Autodesk Inventor part; units mm, degrees
ref_plane "YZ Plane" through (0, 0, 0) normal (1, 0, 0) x (0, 1, 0)
ref_plane "XZ Plane" through (0, 0, 0) normal (0, 1, 0) x (-1, 0, 0)
ref_plane "XY Plane" through (0, 0, 0) normal (0, 0, 1) x (1, 0, 0)
sketch "Эскиз1" plane through (0, 0, 0) normal (0, 0, 1) x (1, 0, 0)
  line L0 (-17.6, 17.6) -> (17.6, 17.6)
  line L1 (17.6, 17.6) -> (17.6, -17.6)
  line L2 (17.6, -17.6) -> (-17.6, -17.6)
  line L3 (-17.6, -17.6) -> (-17.6, 17.6)
  point P0 (13, -13)
  point P1 (-13, -13)
  point P2 (13, 13)
  point P3 (-13, 13)
  dimension "d0" = 35.2
  dimension "d1" = 35.2
extrude "Выдавливание1" add sketch "Эскиз1" along normal blind 26
sketch "Эскиз2" plane through (0, 0, 26) normal (0, 0, 1) x (1, 0, 0)
  circle A0 centre (0, 0) radius 11
  dimension "d6" = 22
extrude "Выдавливание2" add sketch "Эскиз2" along normal blind 2
sketch "Эскиз3" plane through (0, 0, 28) normal (0, 0, 1) x (1, 0, 0)
  circle A0 centre (0, 0) radius 11
  circle A1 centre (0, 0) radius 2.5
  dimension "d9" = 5
extrude "Выдавливание3" add sketch "Эскиз3" along normal blind 22 contours A1
sketch "Эскиз4" plane through (0, 0, 50) normal (0, 0, 1) x (1, 0, 0)
  line L0 (0, 2) -> (3.1194, 2)
  line L1 (3.1194, 2) -> (3.1194, 3.4913)
  line L2 (3.1194, 3.4913) -> (-4.7004, 3.4913)
  line L3 (-4.7004, 3.4913) -> (-4.7004, 2)
  line L4 (-4.7004, 2) -> (0, 2)
extrude "Выдавливание4" cut sketch "Эскиз4" against normal blind 15
hole "Отверстие1" at (13, -13, 0) at (13, 13, 0) at (-13, 13, 0) at (-13, -13, 0) direction (0, 0, 1) diameter 3 end through all
fillet "Сопряжение1" radius 1 4 edges at (-17.6, -17.6, 13) (17.6, -17.6, 13) (17.6, 17.6, 13) (-17.6, 17.6, 13)
properties part number "MotorNema14"
The model under review builds one solid part; all positions refer to its coordinate system, in mm. A direction names the side the tool comes from. Give positions to 0.01 mm unless a question says otherwise; leave off trailing zeros. Write each loop counter-clockwise with the first axis right and the second up, starting at its lowest first coordinate (ties: lowest second). Pieces come first, ordered by that corner, then holes. Notation, with made-up numbers: M -20,59.5 L -6,59.5 A20 ccw -6,91.5 Z; hole C -23.5,17 d8. An arc over 180 degrees is marked long. Write each question's results on one line, items separated by ' | '. Start each with the question number.
1. We need section D-D (y = 0). Write out the cut boundary in (x, z), and give its area (3 significant figures).
2. We need section A-A (x = 13). Write out the cut boundary in (y, z).
3. For probe 1 along Y at (x, z) = (13, 17); probe 2 along Z at (x, y) = (-15, 13.5), list the stretches that pass through material, from the lowest coordinate up. Write a range as [from, to].
4. Insertion check: pin 1 Ø5 at (x, y) = (-13, 13) entering from +Z; pin 2 Ø10.5 at (x, y) = (-2, 6.5) entering from +Z; pin 3 Ø0.6 at (x, y) = (0, 2.5) entering from +Z; pin 4 Ø3 at (x, y) = (11.5, -4) entering from +Z. Each pin has a flat end and moves straight along its axis. Give the tip position at first contact, or say it passes through.
5. For faces 4 (the cylindrical face through (12.93, 11.5, 13.18)), 5 (the cylindrical face through (-2.38, 10.74, 26.99)), list the 3-axis set-ups (+Z, -Z, +X, -X, +Y, -Y) from which the entire face can be reached by the end or side of a thin tool; tool diameter is ignored.
6. Mouldability with a two-part tool opening along X and no side actions: class faces 1 (the cylindrical face through (-0.33, -2.48, 38.85)), 2 (the cylindrical face through (12.93, -14.5, 13.18)), 3 (the flat face through (0, 2, 43)) as released by +X, released by -X, zero draft, split by the parting line, or undercut.
7. We need section C-C (z = 11.5). Write out the cut boundary in (x, y).
Results found:
1) outline: M -17.6,0 L 17.6,0 L 17.6,26 L 11,26 L 11,28 L 2.5,28 L 2.5,50 L -2.5,50 L -2.5,28 L -11,28 L -11,26 L -17.6,26 Z | area: 1,070 mm^2
2) outline: M -17.6,0 L -14.5,0 L -14.5,26 L -17.6,26 Z; M -11.5,0 L 11.5,0 L 11.5,26 L -11.5,26 Z; M 14.5,0 L 17.6,0 L 17.6,26 L 14.5,26 Z
3) probe 1: y = [-17.6, -14.5], [-11.5, 11.5], [14.5, 17.6] | probe 2: z = [0, 26]
4) pin 1: stops at z = 26 | pin 2: stops at z = 50 | pin 3: stops at z = 35 | pin 4: stops at z = 28
5) face 4: +Z, -Z | face 5: +Z
6) face 1: split by the parting line | face 2: undercut | face 3: zero draft
7) outline: M -17.6,-16.6 A1 ccw -16.6,-17.6 L 16.6,-17.6 A1 ccw 17.6,-16.6 L 17.6,16.6 A1 ccw 16.6,17.6 L -16.6,17.6 A1 ccw -17.6,16.6 Z; hole C -13,-13 d3; hole C -13,13 d3; hole C 13,-13 d3; hole C 13,13 d3
